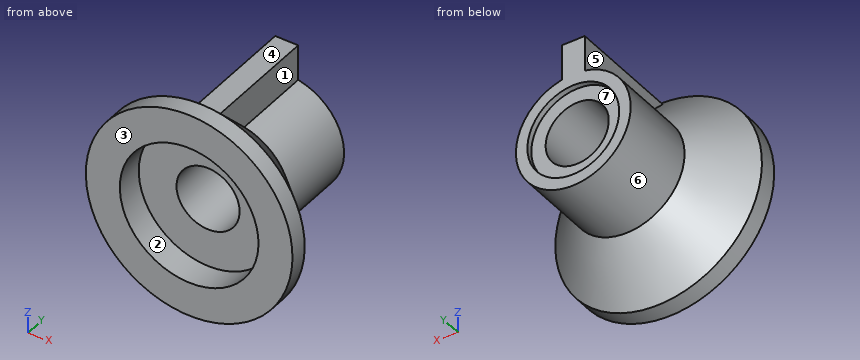
from build123d import *

# Parameters (mm, degrees)
SKETCH2_W           = 2
SKETCH2_H           = 12.5
BOSS_EXTRUDE1_DEPTH = 3.5
SKETCH3_W           = 6.040817985
SKETCH3_H           = 3.31390433


with BuildPart() as part:
    # Sketch1 → Revolve1 (revolve)
    with BuildSketch(Plane(origin=(0, 0, 0), x_dir=(0, 0, -1), z_dir=(1, 0, 0))):
        Polygon((-4, 14.088414634), (-4, 14.588414634), (-5, 14.588414634), (-5, 7.679878049), (-9, 3.655487805), (-9, 2.088414634), (-6, 2.088414634), (-6, 4.509146341), (-2.75, 4.509146341), (-2.75, 14.088414634), align=None)
    revolve(axis=Axis((0, 0, 0), (0, 1, 0)))

    # Sketch2 → Boss-Extrude1 (add)
    with BuildSketch(Plane.XY.offset(8)):
        with Locations((0, 8.338414634)):
            Rectangle(SKETCH2_W, SKETCH2_H)
    extrude(amount=-BOSS_EXTRUDE1_DEPTH)

    # Sketch3 → Cut-Revolve1 (revolve, cut)
    with BuildSketch(Plane(origin=(0, 0, 0), x_dir=(0, 0, -1), z_dir=(1, 0, 0))):
        with Locations((3.020408993, 2.852194176)):
            Rectangle(SKETCH3_W, SKETCH3_H)
    revolve(axis=Axis((0, 1.195242011, 0), (0, 1, 0)), mode=Mode.SUBTRACT)


solid = part.part
Can you work these out from the model? Positions are in its coordinate system, mm. Face numbers are marked on the shaded views. A direction names the side the tool comes from. Round coordinates to 2 decimals unless told otherwise and drop trailing zeros. Write each loop counter-clockwise with the first axis right and the second up, starting at its lowest first coordinate (ties: lowest second). Pieces come first, ordered by that corner, then holes. Notation, with made-up numbers: M -33,33 L -14,33 A23 ccw -14,69 Z; hole C -0.75,47.25 d11. An arc over 180 degrees is marked long. Use a Markdown table: item, result.
Item 1: Which directions (+Z, -Z, +X, -X, +Y, -Y) give clear straight access to the entire face, cutting with the end or side of a thin tool? Please do the marked faces 1, 2, 3 and 4.
Found:
| item | result |
|---|---|
| face 1 | +Z, +X, +Y |
| face 2 | -Y |
| face 3 | +Z, -Z, +X, -X, -Y |
| face 4 | +Z, +X, -X, +Y |
Item 2: I want a section at B-B (z = 0). List the corners of the cut face in (x, y) for me, and give its area (3 significant figures).
Found:
| item | result |
|---|---|
| outline | M -9,2.09 L -6.04,2.09 L -6.04,4.51 L -2.75,4.51 L -2.75,14.09 L -4,14.09 L -4,14.59 L -5,14.59 L -5,7.68 L -9,3.66 Z; M 2.75,4.51 L 6.04,4.51 L 6.04,2.09 L 9,2.09 L 9,3.66 L 5,7.68 L 5,14.59 L 4,14.59 L 4,14.09 L 2.75,14.09 Z |
| area | 67.7 mm2 |
Item 3: I want a section at C-C (x = 0). List the corners of the cut face in (y, z) for me, and give its area (3 significant figures).
Found:
| item | result |
|---|---|
| outline | M 2.09,-9 L 3.66,-9 L 7.68,-5 L 14.59,-5 L 14.59,-4 L 14.09,-4 L 14.09,-2.75 L 4.51,-2.75 L 4.51,-6.04 L 2.09,-6.04 Z; M 2.09,6.04 L 4.51,6.04 L 4.51,2.75 L 14.09,2.75 L 14.09,4 L 14.59,4 L 14.59,8 L 4.66,8 L 3.66,9 L 2.09,9 Z |
| area | 93.0 mm2 |
Item 4: I want a section at D-D (y = 4.25). List the corners of the cut face in (x, z) for me.
Found:
| item | result |
|---|---|
| outline | C 0,0 d16.82; hole C 0,0 d12.08 |
Item 5: For pin 1 Ø4 at (x, z) = (1, -0.5) entering from -Y; pin 2 Ø1.6 at (y, z) = (11.5, 7) entering from -X; pin 3 Ø1.5 at (x, y) = (0, 8) entering from -Z; pin 4 Ø5 at (x, z) = (-4, -2.5) entering from -Y, each with a flat end and sliding along its axis, tell me the tip position at first contact or that it passes through.
Found:
| item | result |
|---|---|
| pin 1 | stops at y = 4.51 |
| pin 2 | stops at x = -1 |
| pin 3 | stops at z = -5.43 |
| pin 4 | stops at y = 2.09 |
Item 6: We'd pull the mould along Z, two halves only. Please class the marked faces 5, 6 and 7: released by +Z, released by -Z, zero draft, split by the parting line, or undercut.
Found:
| item | result |
|---|---|
| face 5 | zero draft |
| face 6 | split by the parting line |
| face 7 | undercut |
Item 7: If I drill on line 1 along X through (y, z) = (14.4, 0); line 2 along X through (y, z) = (8.25, 0); line 3 along Y through (x, z) = (2.25, 3.25), over which ranges is the centre line in solid material (lowest first)? Write a range as [from, to].
Found:
| item | result |
|---|---|
| line 1 | x = [-5, -4], [4, 5] |
| line 2 | x = [-5, -2.75], [2.75, 5] |
| line 3 | y = [4.51, 14.09] |
Item 8: I want a section at A-A (y = 12.5). List the corners of the cut face in (x, z) for me, and give its area (3 significant figures).
Found:
| item | result |
|---|---|
| outline | M -1,4.9 A5 ccw long 1,4.9 L 1,8 L -1,8 Z; hole C 0,0 d5.5 |
| area | 60.8 mm2 |
